Here's how the part is built. I have some questions about the finished solid (model axes, mm). A direction names the side the tool comes from. Round coordinates to 2 decimals unless told otherwise and drop trailing zeros. Loops run counter-clockwise (first coordinate to the right, second up) from the corner with the lowest first, then second, coordinate; pieces in that order, holes last. Notation, with made-up numbers: (-8, -33.75) -> (38, -33.75) arc R19 ccw to (38, -6.75) -> close; hole circle Ø10 at (-15.75, 88.5). An arc over 180 degrees is marked (long way). Use one line per item in the form item = value. Start each with the question number.
Item 1: If we section it at C-C (z = 95): Write out the boundary of the cut face in (x, y), then the cut area to 3 significant figures.
Item 2: For faces 1 (the face through (5, -39, 6)), 2 (the face through (10, -40, 5)), 3 (the face through (0, -43, 95)), 4 (the face through (0, -43, 5)), 5 (the face through (-5.29, -36.77, 102.46)), which set-ups out of +Z, -Z, +X, -X, +Y, -Y let a thin tool reach every point of the face, with its end or its side?
Item 3: If we section it at D-D (x = 5): Write out the boundary of the cut face in (y, z), then the cut area to 3 significant figures.
Item 4: Thinking about a two-plate mould opening in Y: for faces 6 (the face through (4.71, -41.23, 2.96)), 7 (the face through (0, -36, 100)), 8 (the face through (4.71, -36.77, 102.46)), which applies, released by +Y, released by -Y, zero draft, split by the parting line, or undercut?
Item 5: If we section it at A-A (y = -28.5): Write out the boundary of the cut face in (x, z), then the cut area to 3 significant figures.
Item 6: If we section it at B-B (x = 28): Write out the boundary of the cut face in (y, z).
Item 7: If I drill on L1, parallel to X at y = -39, z = 1; L2, parallel to X at y = -53.5, z = 53; L3, parallel to X at y = -25, z = 30, over which ranges is the centre line in solid material (lowest first)? Write a range as [from, to].
Item 8: I'm going to push flat-ended pins straight in: pin 1 Ø2 at (x, y) = (-5.5, -39) entering from -Z; pin 2 Ø11.5 at (y, z) = (-60.5, 53) entering from -X; pin 3 Ø3 at (y, z) = (-29, 84.5) entering from -X. Where does each tip first touch, or does it pass through?
```python
from build123d import *

# Parameters (mm, degrees)
EXTRUDE_THIN1_DEPTH       = 100
BOSS_EXTRUDE1_START       = -10
BOSS_EXTRUDE1_DEPTH       = 10
SKETCH3_R                 = 2.25
BOSS_EXTRUDE2_DEPTH       = 5
BOSS_EXTRUDE3_DEPTH       = 10
SKETCH5_R                 = 2.25
CUT_EXTRUDE1_DEPTH        = 6
BOSS_EXTRUDE4_REACH       = 121.416
BOSS_EXTRUDE4_END_RADIUS  = 39
SKETCH10_W                = 20
SKETCH10_H                = 20
BOSS_EXTRUDE5_START       = -26.86522245
BOSS_EXTRUDE5_OUTLINE_W   = 20
BOSS_EXTRUDE5_OUTLINE_H   = 20
BOSS_EXTRUDE5_DEPTH       = 26.86522245
BOSS_EXTRUDE5_START_2     = 78.671989238
BOSS_EXTRUDE5_2_OUTLINE_W = 23
BOSS_EXTRUDE5_2_OUTLINE_H = 23
BOSS_EXTRUDE5_2_DEPTH     = 3.328010762
BOSS_EXTRUDE6_DEPTH       = 20
SKETCH12_R                = 2.5
CUT_EXTRUDE2_DEPTH        = 20


with BuildPart() as part:
    # Sketch1 → Extrude-Thin1 (new body)
    with BuildSketch(Plane.XY):
        with BuildLine():
            ThreePointArc((-35, 0), (0, -35), (35, 0))
            Line((35, 0), (39, 0))
            ThreePointArc((39, 0), (0, -39), (-39, 0))
            Line((-39, 0), (-35, 0))
        make_face()
    extrude(amount=EXTRUDE_THIN1_DEPTH)

    # Sketch2 → Boss-Extrude1 (add)
    with BuildSketch(Plane.XY.offset(100).offset(BOSS_EXTRUDE1_START)):
        with BuildLine():
            Line((0, -39), (0, -35))
            Line((0, -35), (-10, -35))
            Line((-10, -35), (-10, -37.69615365))
            ThreePointArc((-10, -37.69615365), (-5.042321274, -38.672664715), (0, -39))
        make_face()
        with BuildLine():
            Line((10, -35), (0, -35))
            Line((0, -35), (0, -39))
            ThreePointArc((0, -39), (5.042321274, -38.672664715), (10, -37.69615365))
            Line((10, -37.69615365), (10, -35))
        make_face()
        with BuildLine():
            ThreePointArc((10, -37.69615365), (5.042321274, -38.672664715), (0, -39))
            ThreePointArc((0, -39), (-5.042321274, -38.672664715), (-10, -37.69615365))
            Line((-10, -37.69615365), (-10, -43))
            Line((-10, -43), (10, -43))
            Line((10, -43), (10, -37.69615365))
        make_face()
    extrude(amount=BOSS_EXTRUDE1_DEPTH)

    # Sketch3 → Boss-Extrude2 (add)
    with BuildSketch(Plane.XY.offset(100)):
        with Locations((-5, -39)):
            Circle(SKETCH3_R)
        with Locations((5, -39)):
            Circle(SKETCH3_R)
    extrude(amount=BOSS_EXTRUDE2_DEPTH)

    # Sketch4 → Boss-Extrude3 (add)
    with BuildSketch(Plane(origin=(0, 0, 0), x_dir=(-1, 0, 0), z_dir=(0, 0, -1))):
        with BuildLine():
            Line((0, -39), (0, -35))
            Line((0, -35), (-10, -35))
            Line((-10, -35), (-10, -37.69615365))
            ThreePointArc((-10, -37.69615365), (-5.042321274, -38.672664715), (0, -39))
        make_face()
        with BuildLine():
            ThreePointArc((10, -37.69615365), (5.042321274, -38.672664715), (0, -39))
            ThreePointArc((0, -39), (-5.042321274, -38.672664715), (-10, -37.69615365))
            Line((-10, -37.69615365), (-10, -43))
            Line((-10, -43), (10, -43))
            Line((10, -43), (10, -37.69615365))
        make_face()
        with BuildLine():
            Line((10, -35), (0, -35))
            Line((0, -35), (0, -39))
            ThreePointArc((0, -39), (5.042321274, -38.672664715), (10, -37.69615365))
            Line((10, -37.69615365), (10, -35))
        make_face()
    extrude(amount=-BOSS_EXTRUDE3_DEPTH)

    # Sketch5 → Cut-Extrude1 (cut)
    with BuildSketch(Plane(origin=(0, 0, 0), x_dir=(-1, 0, 0), z_dir=(0, 0, -1))):
        with Locations(Location((-5, -39, 0), (0, 0, 180))):
            Circle(SKETCH5_R)
        with Locations(Location((5, -39, 0), (0, 0, 180))):
            Circle(SKETCH5_R)
    extrude(amount=-CUT_EXTRUDE1_DEPTH, mode=Mode.SUBTRACT)

    # Boss-Extrude4: up to this cylinder (the profile starts outside it)
    boss_extrude4_end = Plane(origin=(0, 0, 50), z_dir=(0, 0, -1)) * Cylinder(BOSS_EXTRUDE4_END_RADIUS, 321.832, mode=Mode.PRIVATE)
    # Sketch10 → Boss-Extrude4 (add, up to the surface)
    with BuildSketch(Plane(origin=(0, -51.355775573, 4.493048169), x_dir=(1, 0, 0), z_dir=(0, 0.9961946980917462, -0.08715574274765152)), mode=Mode.PRIVATE) as boss_extrude4_sk1:
        with Locations((0, -45.680780994)):
            Rectangle(SKETCH10_W, SKETCH10_H)
    boss_extrude4_tool1 = extrude(boss_extrude4_sk1.sketch, amount=BOSS_EXTRUDE4_REACH, mode=Mode.PRIVATE) - boss_extrude4_end
    add(boss_extrude4_tool1.solids().sort_by_distance((0, -47.374433, 50))[0])

    # Boss-Extrude5: read off the stored shape, not the designer's step
    # Boss-Extrude5 outline → Boss-Extrude5 (add)
    with BuildSketch(Plane(origin=(0, -51.355775573, 4.493048169), x_dir=(1, 0, 0), z_dir=(0, 0.9961946980917462, -0.08715574274765152)).offset(BOSS_EXTRUDE5_START)):
        with Locations((0, -45.680780994)):
            Rectangle(BOSS_EXTRUDE5_OUTLINE_W, BOSS_EXTRUDE5_OUTLINE_H)
    extrude(amount=BOSS_EXTRUDE5_DEPTH)

    # Boss-Extrude5 2 outline → Boss-Extrude5 2 (cut)
    with BuildSketch(Plane(origin=(0, 0, 0), x_dir=(0.9966522374056315, 0.0811043240761468, -0.010315342480997098), z_dir=(0.08175767654690848, -0.9886876617314986, 0.12574732548071493)).offset(BOSS_EXTRUDE5_START_2)):
        with Locations((-6.5, 42.5)):
            Rectangle(BOSS_EXTRUDE5_2_OUTLINE_W, BOSS_EXTRUDE5_2_OUTLINE_H)
    extrude(amount=BOSS_EXTRUDE5_2_DEPTH, mode=Mode.SUBTRACT)

    # Sketch11 → Boss-Extrude6 (add, along a direction that is not the sketch's normal)
    with BuildSketch(Plane(origin=(10, 0, 0), x_dir=(0, 0, -1), z_dir=(1, 0, 0))):
        Polygon((-42.236409552, -73.373320758), (-41.361522917, -63.373320758), (-61.216981199, -60.847982502), (-62.091867834, -70.847982502), align=None)
    extrude(amount=BOSS_EXTRUDE6_DEPTH, dir=(0.9966471031139101, 0.08150889038642521, -0.007131103885419538))

    # Sketch12 → Cut-Extrude2 (cut)
    with BuildSketch(Plane(origin=(5.614716446, -67.898222027, 8.635709896), x_dir=(0.9966522374056316, 0.0811043240761468, -0.010315342480997105), z_dir=(-0.08175767654690848, 0.9886876617314987, -0.12574732548071463))):
        with Locations(Location((14.399910724, -38.067319735, 0), (0, 0, 270))):
            Circle(SKETCH12_R)
        with Locations(Location((14.399910724, -48.082676206, 0), (0, 0, 270))):
            Circle(SKETCH12_R)
    extrude(amount=-CUT_EXTRUDE2_DEPTH, mode=Mode.SUBTRACT)


solid = part.part
```
Values found:
q1.outline = (-39, 0) arc R39 ccw to (-10, -37.7) -> (-10, -43) -> (10, -43) -> (10, -37.7) arc R39 ccw to (39, 0) -> (35, 0) arc R35 cw to (-35, 0) -> close
q1.area = 554 mm2
q2.face_1 = -Z
q2.face_2 = +Z, -Z, +X, -Y
q2.face_3 = +Z, +X, -X, -Y
q2.face_4 = -Z, +X, -X, -Y
q2.face_5 = +Z
q3.outline = (-73.78, 42.27) -> (-38.68, 39.2) -> (-38.68, 10) -> (-43, 10) -> (-43, 0) -> (-41.25, 0) -> (-41.25, 6) -> (-36.75, 6) -> (-36.75, 0) -> (-34.64, 0) -> (-34.64, 100) -> (-36.75, 100) -> (-36.75, 105) -> (-41.25, 105) -> (-41.25, 100) -> (-43, 100) -> (-43, 90) -> (-38.68, 90) -> (-38.68, 59.28) -> (-71.26, 62.13) -> close
q3.area = 1,170 mm2
q4.face_6 = undercut
q4.face_7 = zero draft
q4.face_8 = split by the parting line
q5.outline = (-26.62, 0) -> (-20.32, 0) -> (-20.32, 100) -> (-26.62, 100) -> close; (20.32, 0) -> (26.62, 0) -> (26.62, 100) -> (20.32, 100) -> close
q5.area = 1,260 mm2
q6.outline = (-71.9, 42.11) -> (-61.9, 41.23) -> (-59.38, 61.09) -> (-69.38, 61.96) -> close; (-27.15, 0) -> (-21, 0) -> (-21, 100) -> (-27.15, 100) -> close
q7.L1 = [-10, -7.25], [-2.75, 2.75], [7.25, 10]
q7.L2 = [-10, 10]
q7.L3 = [-29.93, -24.49], [24.49, 29.93]
q8.pin_1 = 6
q8.pin_2 = -10
q8.pin_3 = -27.65
